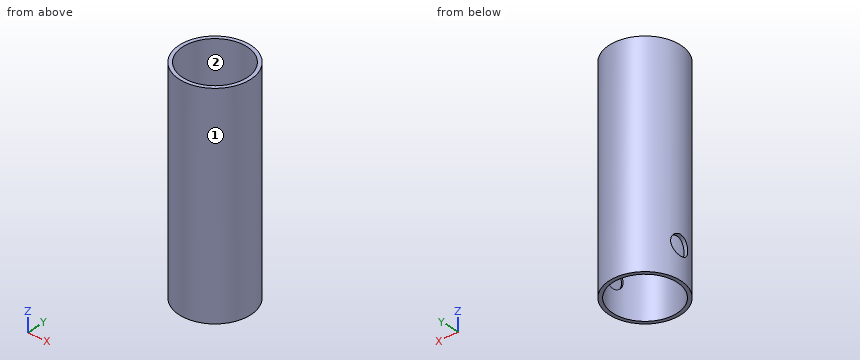
```python
from build123d import *

# Parameters (mm, degrees)
F0_R          = 10
F0_R_2        = 9
F1_DEPTH      = 30
F2_R          = 2.75
F3_DEPTH      = 25
F3_DEPTH_BACK = 9


with BuildPart() as f1:
    # F0 (on Top) → F1 (new body, symmetric)
    with BuildSketch(Plane.XY):
        Circle(F0_R)
        Circle(F0_R_2, mode=Mode.SUBTRACT)
    extrude(amount=F1_DEPTH, both=True)

    # F2 (on Right) → F3 (cut, two sides)
    with BuildSketch(Plane.YZ) as f3_sk:
        with Locations((0, -21)):
            Circle(F2_R)
    extrude(amount=-F3_DEPTH, mode=Mode.SUBTRACT)
    extrude(f3_sk.sketch, amount=F3_DEPTH_BACK, mode=Mode.SUBTRACT)


solid = f1.part
```
Source: CAD feature listing. Evaluate the final solid. Frame: model axes, mm. Face numbers are marked on the shaded views. Coordinates: 2 decimals unless noted, no trailing zeros. Order: outer loops, then holes, each group sorted by start corner. A loop starts at its lowest first (then second) coordinate and runs counter-clockwise, first axis right, second up. Notation, with made-up numbers: (-13.5, 16.25) - (26.5, 16.25) arc R21 cw to (26.5, 54.25) - close; hole circle Ø11 at (40.25, 63.5). An arc over 180 degrees is marked (long way). One line per item, written item: value.
1) Mould query, pull axis X, two halves, no side actions, for the marked faces 1 and 2. Classes: released by +X, released by -X, zero draft, split by the parting line, or undercut.
Computed values:
face 1: split by the parting line
face 2: undercut
2) Cut plane A-A on x = 0. Output: boundary loops of the cut face in (y, z).
Computed values:
outline: (-10, -30) - (-9, -30) - (-9, 30) - (-10, 30) - close; (9, -30) - (10, -30) - (10, 30) - (9, 30) - close
3) Cut plane B-B on y = 7.25. Output: boundary loops of the cut face in (x, z).
Computed values:
outline: (-6.89, -30) - (-5.33, -30) - (-5.33, 30) - (-6.89, 30) - close; (5.33, -30) - (6.89, -30) - (6.89, 30) - (5.33, 30) - close
4) Cut plane C-C on z = 4. Output: boundary loops of the cut face in (x, y), plus the area to 3 significant figures.
Computed values:
outline: circle Ø20 at (0, 0); hole circle Ø18 at (0, 0)
area: 59.7 mm^2
5) Contact query for flat-ended pins moving along their axis: pin 1 (12 mm diameter, centred on x = -2, y = -2, fed in from +Z); pin 2 (1 mm diameter, centred on y = -3, z = 12.5, fed in from +X); pin 3 (3 mm diameter, centred on y = 4.5, z = -17.5, fed in from -X); pin 4 (1 mm diameter, centred on y = -2.5, z = -13, fed in from +X). Output: stop coordinate, or through.
Computed values:
pin 1: passes through
pin 2: stops at x = 9.68
pin 3: stops at x = -9.54
pin 4: stops at x = 9.8
6) Ray query, line 1 (X direction, y = 0, z = 8.5); line 2 (X direction, y = -2.25, z = 1). Return the intervals inside material, ascending. Write a range as [from, to].
Computed values:
line 1: x = [-10, -9], [9, 10]
line 2: x = [-9.74, -8.71], [8.71, 9.74]
7) Cut plane D-D on z = -21. Output: boundary loops of the cut face in (x, y), plus the area to 3 significant figures.
Computed values:
outline: (-9.61, -2.75) arc R10 ccw (long way) to (-9.61, 2.75) - (-8.57, 2.75) arc R9 cw to (8.57, 2.75) - (9, 2.75) - (9, -2.75) - (8.57, -2.75) arc R9 cw to (-8.57, -2.75) - close
area: 53.3 mm^2
